```python
from build123d import *

# Parameters (mm, degrees)
SKETCH1_R           = 75
BOSS_EXTRUDE1_DEPTH = 100
SKETCH3_R           = 37.5
BOSS_EXTRUDE2_DEPTH = 250
SKETCH4_R           = 62.5
BOSS_EXTRUDE3_DEPTH = 75
SKETCH5_W           = 50
SKETCH5_H           = 75
BOSS_EXTRUDE4_DEPTH = 10
SKETCH6_W           = 10
SKETCH6_H           = 75
BOSS_EXTRUDE5_DEPTH = 70
SKETCH7_R           = 7.5
BOSS_EXTRUDE6_DEPTH = 40
BOSS_EXTRUDE7_START = 61
SKETCH8_R           = 32.966655639
SKETCH8_R_2         = 7.5
BOSS_EXTRUDE7_DEPTH = 61
CHAMFER2_SIZE       = 7
BOSS_EXTRUDE8_START = 30
SKETCH9_R           = 12
SKETCH9_R_2         = 7.5
BOSS_EXTRUDE8_DEPTH = 30
FILLET1_R           = 30
CHAMFER4_SIZE       = 10
CHAMFER5_START      = 353
CHAMFER5_OUTLINE_W  = 21
CHAMFER5_OUTLINE_H  = 25
CHAMFER5_DEPTH      = 9.287293916
CHAMFER6_START      = 353
CHAMFER6_OUTLINE_W  = 21
CHAMFER6_OUTLINE_H  = 25
CHAMFER6_DEPTH      = 9.287293916
CHAMFER7_START      = -362.287293916
CHAMFER7_OUTLINE_W  = 21
CHAMFER7_OUTLINE_H  = 25
CHAMFER7_DEPTH      = 9.287293916
CHAMFER8_START      = -362.287293916
CHAMFER8_OUTLINE_W  = 21
CHAMFER8_OUTLINE_H  = 25
CHAMFER8_DEPTH      = 9.287293916
SKETCH10_R          = 67.5
BOSS_EXTRUDE9_DEPTH = 10


with BuildPart() as part:
    # Sketch1 → Boss-Extrude1 (new body)
    with BuildSketch(Plane.XY):
        Circle(SKETCH1_R)
    extrude(amount=BOSS_EXTRUDE1_DEPTH)

    # Loft1: read off the stored shape, not the designer's step
    # Loft1: loft between two sections, ruled curve by curve
    loft1_from = [
        Edge.make_bspline([(55.013686164, 50.975428734, 100), (-46.937171304, 161.002801063, 100), (-156.964543632, 59.051943595, 100), (-55.013686164, -50.975428734, 100), (46.937171304, -161.002801063, 100), (156.964543632, -59.051943595, 100), (55.013686164, 50.975428734, 100)], [0, 0, 0, 0, 0.5, 0.5, 0.5, 1, 1, 1, 1], 3, [1, 0.333333333, 0.333333333, 1, 0.333333333, 0.333333333, 1]),
    ]
    loft1_to = [
        Edge.make_bspline([(-15.510833372, 34.141822566, 450), (-83.794478503, 3.120155821, 450), (-52.772811759, -65.16348931, 450), (15.510833372, -34.141822566, 450), (83.794478503, -3.120155821, 450), (52.772811759, 65.16348931, 450), (-15.510833372, 34.141822566, 450)], [0, 0, 0, 0, 0.5, 0.5, 0.5, 1, 1, 1, 1], 3, [1, 0.333333333, 0.333333333, 1, 0.333333333, 0.333333333, 1]),
    ]
    loft1 = Solid(Shell([*[Face.make_surface_from_curves(loft1_from[k], loft1_to[k]) for k in range(1)], Face(Wire(loft1_from)), Face(Wire(loft1_to))]))
    add(loft1)

    # Sketch3 → Boss-Extrude2 (add)
    with BuildSketch(Plane.XY.offset(450)):
        with Locations(Location((0, 0, 0), (0, 0, 114.432581244))):
            Circle(SKETCH3_R)
    extrude(amount=BOSS_EXTRUDE2_DEPTH)

    # Sketch4 → Boss-Extrude3 (add)
    with BuildSketch(Plane(origin=(0, 0, 0), x_dir=(-1, 0, 0), z_dir=(0, 0, -1))):
        Circle(SKETCH4_R)
    extrude(amount=BOSS_EXTRUDE3_DEPTH)

    # Sketch5 → Boss-Extrude4 (add)
    with BuildSketch(Plane.XY.offset(700)):
        with Locations((-25, 0)):
            Rectangle(SKETCH5_W, SKETCH5_H)
    boss_extrude4 = extrude(amount=BOSS_EXTRUDE4_DEPTH)

    # Sketch6 → Boss-Extrude5 (add)
    with BuildSketch(Plane.XY.offset(710)):
        with Locations((-45, 0)):
            Rectangle(SKETCH6_W, SKETCH6_H)
    boss_extrude5 = extrude(amount=BOSS_EXTRUDE5_DEPTH)

    # Sketch7 → Boss-Extrude6 (add)
    with BuildSketch(Plane(origin=(-40, 0, 0), x_dir=(0, 0, -1), z_dir=(1, 0, 0))):
        with Locations(Location((-745, 0, 0), (0, 0, 270))):
            Circle(SKETCH7_R)
    boss_extrude6 = extrude(amount=BOSS_EXTRUDE6_DEPTH)

    # Mirror1: Boss-Extrude4, Boss-Extrude5, Boss-Extrude6 across plane
    add(boss_extrude4.mirror(Plane(origin=(0, 0, 710), x_dir=(0, 0, 1), z_dir=(-1, 0, 0))))
    add(boss_extrude5.mirror(Plane(origin=(0, 0, 710), x_dir=(0, 0, 1), z_dir=(-1, 0, 0))))
    add(boss_extrude6.mirror(Plane(origin=(0, 0, 710), x_dir=(0, 0, 1), z_dir=(-1, 0, 0))))

    # Sketch8 → Boss-Extrude7 (add)
    # profile 1 of 2: a face of its own
    with BuildSketch(Plane.ZY.offset(50).offset(BOSS_EXTRUDE7_START)):
        with Locations(Location((745, 0, 0), (0, 0, 180))):
            Circle(SKETCH8_R)
        with Locations(Location((745, 0, 0), (0, 0, 270))):
            Circle(SKETCH8_R_2, mode=Mode.SUBTRACT)
    # profile 2 of 2: a face of its own
    with BuildSketch(Plane.ZY.offset(50).offset(BOSS_EXTRUDE7_START)):
        with Locations(Location((745, 0, 0), (0, 0, 270))):
            Circle(SKETCH8_R_2)
    extrude(amount=-BOSS_EXTRUDE7_DEPTH)

    # Chamfer2
    chamfer2_edges = [part.edges().sort_by_distance(p)[0] for p in [
        (-111, 0, 777.966655639),
    ]]
    chamfer(chamfer2_edges, length=CHAMFER2_SIZE)

    # Sketch9 → Boss-Extrude8 (add)
    with BuildSketch(Plane.ZY.offset(-40).offset(BOSS_EXTRUDE8_START)):
        with Locations(Location((745, 0, 0), (0, 0, 270))):
            Circle(SKETCH9_R)
        with Locations(Location((745, 0, 0), (0, 0, 270))):
            Circle(SKETCH9_R_2, mode=Mode.SUBTRACT)
    boss_extrude8 = extrude(amount=-BOSS_EXTRUDE8_DEPTH)

    # Mirror2: Boss-Extrude8 across plane
    add(boss_extrude8.mirror(Plane(origin=(0, 0, 0), x_dir=(0, 0, 1), z_dir=(1, 0, 0))))

    # Fillet1
    fillet1_edges = [part.edges().sort_by_distance(p)[0] for p in [
        (-45, -37.5, 780),
        (-45, 37.5, 780),
        (45, 37.5, 780),
        (45, -37.5, 780),
    ]]
    fillet(fillet1_edges, radius=FILLET1_R)

    # Chamfer4
    chamfer4_edges = [part.edges().sort_by_distance(p)[0] for p in [
        (-40, 0, 710),
        (40, 0, 710),
    ]]
    chamfer(chamfer4_edges, length=CHAMFER4_SIZE)

    # Chamfer5: read off the stored shape, not the designer's step
    # Chamfer5 outline → Chamfer5 (cut)
    with BuildSketch(Plane(origin=(0, 0, 0), x_dir=(0.8164965809277258, 0.40824829046386313, -0.40824829046386313), z_dir=(0.5773502691896258, -0.5773502691896258, 0.5773502691896258)).offset(CHAMFER5_START)):
        with Locations((-308.5, 521.5)):
            Rectangle(CHAMFER5_OUTLINE_W, CHAMFER5_OUTLINE_H)
    extrude(amount=CHAMFER5_DEPTH, mode=Mode.SUBTRACT)

    # Chamfer6: read off the stored shape, not the designer's step
    # Chamfer6 outline → Chamfer6 (cut)
    with BuildSketch(Plane(origin=(0, 0, 0), x_dir=(0.8164965809277258, -0.40824829046386313, -0.40824829046386313), z_dir=(0.5773502691896258, 0.5773502691896258, 0.5773502691896258)).offset(CHAMFER6_START)):
        with Locations((-308.5, -521.5)):
            Rectangle(CHAMFER6_OUTLINE_W, CHAMFER6_OUTLINE_H)
    extrude(amount=CHAMFER6_DEPTH, mode=Mode.SUBTRACT)

    # Chamfer7: read off the stored shape, not the designer's step
    # Chamfer7 outline → Chamfer7 (cut)
    with BuildSketch(Plane(origin=(0, 0, 0), x_dir=(0.8164965809277258, -0.40824829046386313, 0.40824829046386313), z_dir=(0.5773502691896258, 0.5773502691896258, -0.5773502691896258)).offset(CHAMFER7_START)):
        with Locations((308.5, -521.5)):
            Rectangle(CHAMFER7_OUTLINE_W, CHAMFER7_OUTLINE_H)
    extrude(amount=CHAMFER7_DEPTH, mode=Mode.SUBTRACT)

    # Chamfer8: read off the stored shape, not the designer's step
    # Chamfer8 outline → Chamfer8 (cut)
    with BuildSketch(Plane(origin=(0, 0, 0), x_dir=(0.8164965809277258, 0.40824829046386313, 0.40824829046386313), z_dir=(0.5773502691896258, -0.5773502691896258, -0.5773502691896258)).offset(CHAMFER8_START)):
        with Locations((308.5, 521.5)):
            Rectangle(CHAMFER8_OUTLINE_W, CHAMFER8_OUTLINE_H)
    extrude(amount=CHAMFER8_DEPTH, mode=Mode.SUBTRACT)

    # Sketch10 → Boss-Extrude9 (add)
    with BuildSketch(Plane(origin=(0, 0, -75), x_dir=(-1, 0, 0), z_dir=(0, 0, -1))):
        Circle(SKETCH10_R)
    extrude(amount=-BOSS_EXTRUDE9_DEPTH)


solid = part.part
```
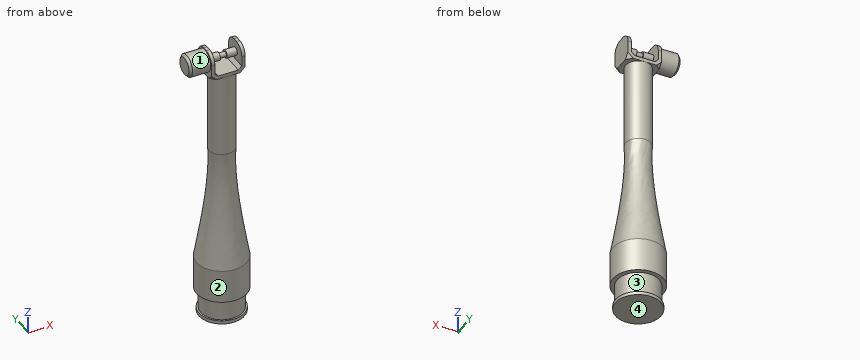
Source: CAD feature listing. Evaluate the final solid. Frame: model axes, mm. Face numbers are marked on the shaded views. Round coordinates to 2 decimals unless told otherwise and drop trailing zeros. Write each loop counter-clockwise with the first axis right and the second up, starting at its lowest first coordinate (ties: lowest second). Pieces come first, ordered by that corner, then holes. Notation, with made-up numbers: M 12.5,58 L 43.5,58 A30 ccw 43.5,84 Z; hole C 28,85 d5. An arc over 180 degrees is marked long. Answer as a JSON object with one key per item and string values. Group by question number.
(1) Ray query, line 1 (Z direction, x = -32, y = 1); line 2 (Z direction, x = 26, y = -22.5); line 3 (Y direction, x = -68, z = 745.5). Return the intervals inside material, ascending. Write a range as [from, to].
(2) Mould query, pull axis Z, two halves, no side actions, for the marked faces 1, 2, 3 and 4. Classes: +Z half, -Z half, draft (parallel to the pull), parting line (faces both ways), or undercut.
(3) Section query A-A on z = 688. Output: boundary loops of the cut face in (x, y).
(4) First-contact query: pin 1 (8 mm diameter, centred on x = -38.5, z = 537, fed in from +Y); pin 2 (5 mm diameter, centred on y = -3, z = 512.5, fed in from +X); pin 3 (12 mm diameter, centred on y = -36.5, z = 305, fed in from -X). Flat tips, straight axial feed; report the tip coordinate or a pass-through.
Computed values:
{
 "1": {"line 1": "[-75, 712], [733.04, 756.96]", "line 2": "[-75, 710]", "line 3": "[-32.96, 32.96]"},
 "2": {"face 1": "undercut", "face 2": "draft", "face 3": "undercut", "face 4": "-Z half"},
 "3": {"outline": "C 0,0 d75"},
 "4": {"pin 1": "y = 14.7", "pin 2": "x = 37.5", "pin 3": "x = -30.86"}
}
